Source: CAD feature listing. Evaluate the final solid. Frame: model axes, mm. Face numbers are marked on the shaded views. A direction names the side the tool comes from. Give positions to 0.01 mm unless a question says otherwise; leave off trailing zeros. Write each loop counter-clockwise with the first axis right and the second up, starting at its lowest first coordinate (ties: lowest second). Pieces come first, ordered by that corner, then holes. Notation, with made-up numbers: (31, 5.25) -> (51, 5.25) arc R24 ccw to (51, 26.25) -> close; hole circle Ø2 at (34.5, 43). An arc over 180 degrees is marked (long way). Answer as a JSON object with one key per item and string values. Group by question number.
Item 1: Section query A-A on x = -45. Return the cut outline in (y, z), plus the area to 3 significant figures.
Item 2: Access query for the marked faces 1 and 2. Directions: +Z, -Z, +X, -X, +Y, -Y. A direction counts if a zero-diameter tool reaches every point of the face in a straight line with its end or side. Return the directions, or none.
Item 3: Section query C-C on y = 2.25. Give the number of separate pieces and of enclosed holes in the cut face, plus the area to 3 significant figures.
Item 4: First-contact query: pin 1 Ø5.5 at (x, z) = (54.28, 54.28) entering from -Y; pin 2 Ø4.5 at (x, z) = (-54.28, 54.28) entering from +Y; pin 3 Ø2 at (y, z) = (0.5, 50) entering from +X. Flat tips, straight axial feed; report the tip coordinate or a pass-through.
Item 5: Section query B-B on z = -12.5. Return the cut outline in (x, y), plus the area to 3 significant figures.
Item 6: Ray query, probe 1 along X at (y, z) = (0.35, 0); probe 2 along Y at (x, z) = (-64.5, -46.5). Return the intervals inside material, ascending. Write a range as from..to.
from build123d import *
from build123d.topology import SkipClean

# Parameters (mm, degrees)
ESBO_O1_R                                    = 82.26
ESBO_O1_R_2                                  = 70
RESSALTO_EXTRUS_O1_DEPTH                     = 3
RESSALTO_EXTRUS_O2_START                     = 1.3
ESBO_O2_R                                    = 73
ESBO_O2_R_2                                  = 70
RESSALTO_EXTRUS_O2_DEPTH                     = 1.3
ESCAREADO_PARA_PARAFUSO_ALLEN_SEXTAV_2_COUNT = 2
ESCAREADO_PARA_PARAFUSO_ALLEN_SEXTAV_2_PITCH = 76.76
ESCAREADO_PARA_PARAFUSO_ALLEN_SEXTAV_3_COUNT = 2
ESCAREADO_PARA_PARAFUSO_ALLEN_SEXTAV_3_PITCH = 76.76
ESCAREADO_PARA_PARAFUSO_ALLEN_SEXTAV_4_COUNT = 2
ESCAREADO_PARA_PARAFUSO_ALLEN_SEXTAV_4_PITCH = 76.76
ESCAREADO_PARA_PARAFUSO_ALLEN_SEXTAV_5_COUNT = 2
ESCAREADO_PARA_PARAFUSO_ALLEN_SEXTAV_5_PITCH = 76.76
ESCAREADO_PARA_PARAFUSO_ALLEN_SEXTAV_6_COUNT = 2
ESCAREADO_PARA_PARAFUSO_ALLEN_SEXTAV_6_PITCH = 76.76
ESCAREADO_PARA_PARAFUSO_ALLEN_SEXTAV_7_COUNT = 2
ESCAREADO_PARA_PARAFUSO_ALLEN_SEXTAV_7_PITCH = 76.76
ESCAREADO_PARA_PARAFUSO_ALLEN_SEXTAV_8_COUNT = 2
ESCAREADO_PARA_PARAFUSO_ALLEN_SEXTAV_8_PITCH = 76.76
ESCAREADO_PARA_PARAFUSO_ALLEN_SEXTAV_9_COUNT = 2
ESCAREADO_PARA_PARAFUSO_ALLEN_SEXTAV_9_PITCH = 76.76
RESSALTO_EXTRUS_O3_START                     = -3
RESSALTO_EXTRUS_O3_DEPTH                     = 3
FILETE1_R                                    = 2
ESBO_O9_R                                    = 1.8
CORTE_EXTRUS_O3_DEPTH                        = 122.035496877
CHANFRO2_SIZE                                = 1


with BuildPart() as part:
    # Esboço1 → Ressalto-extrusão1 (new body)
    with BuildSketch(Plane(origin=(0, 0, 0), x_dir=(1, 0, 0), z_dir=(0, 1, 0))):
        with Locations(Location((0, 0, 0), (0, 0, 270))):
            Circle(ESBO_O1_R)
        with Locations(Location((0, 0, 0), (0, 0, 270))):
            Circle(ESBO_O1_R_2, mode=Mode.SUBTRACT)
    extrude(amount=RESSALTO_EXTRUS_O1_DEPTH)

    # Esboço2 → Ressalto-extrusão2 (add)
    with SkipClean():  # the faces are left unmerged after this step: merging them gives an invalid solid
        with BuildSketch(Plane.XZ.offset(RESSALTO_EXTRUS_O2_START)):
            with Locations(Location((0, 0, 0), (0, 0, 270))):
                Circle(ESBO_O2_R)
            with Locations(Location((0, 0, 0), (0, 0, 270))):
                Circle(ESBO_O2_R_2, mode=Mode.SUBTRACT)
        extrude(amount=-RESSALTO_EXTRUS_O2_DEPTH)

    # Esboço4 → Escareado para parafuso Allen sextavado escareado de M31 (revolve, cut)
    with SkipClean():  # the faces are left unmerged after this step: merging them gives an invalid solid
        with BuildSketch(Plane(origin=(0, 3, 0), x_dir=(0, 0, 1), z_dir=(1, 0, 0))):
            Polygon((0, 0), (0, 3), (1.7, 3), (1.7, 1.66), (3.36, 0), align=None)
        escareado_para_parafuso_allen_sextavado = revolve(axis=Axis((0, 9.35, 0), (0, -1, 0)), mode=Mode.SUBTRACT)

    # Escareado para parafuso Allen sextav 2: Escareado para parafuso Allen sextavado escareado de M31 ×2
    with SkipClean():  # the faces are left unmerged after this step: merging them gives an invalid solid
        with Locations(*[(-i * ESCAREADO_PARA_PARAFUSO_ALLEN_SEXTAV_2_PITCH, 0, 0) for i in range(1, ESCAREADO_PARA_PARAFUSO_ALLEN_SEXTAV_2_COUNT)]):
            add(escareado_para_parafuso_allen_sextavado, mode=Mode.SUBTRACT)

    # Escareado para parafuso Allen sextav 3: Escareado para parafuso Allen sextavado escareado de M31 ×2
    with SkipClean():  # the faces are left unmerged after this step: merging them gives an invalid solid
        with Locations(*[Vector(-0.7071067811865477, 0, -0.7071067811865475) * (i * ESCAREADO_PARA_PARAFUSO_ALLEN_SEXTAV_3_PITCH) for i in range(1, ESCAREADO_PARA_PARAFUSO_ALLEN_SEXTAV_3_COUNT)]):
            add(escareado_para_parafuso_allen_sextavado, mode=Mode.SUBTRACT)

    # Escareado para parafuso Allen sextav 4: Escareado para parafuso Allen sextavado escareado de M31 ×2
    with SkipClean():  # the faces are left unmerged after this step: merging them gives an invalid solid
        with Locations(*[(0, 0, -i * ESCAREADO_PARA_PARAFUSO_ALLEN_SEXTAV_4_PITCH) for i in range(1, ESCAREADO_PARA_PARAFUSO_ALLEN_SEXTAV_4_COUNT)]):
            add(escareado_para_parafuso_allen_sextavado, mode=Mode.SUBTRACT)

    # Escareado para parafuso Allen sextav 5: Escareado para parafuso Allen sextavado escareado de M31 ×2
    with SkipClean():  # the faces are left unmerged after this step: merging them gives an invalid solid
        with Locations(*[Vector(0.7071067811865475, 0, -0.7071067811865476) * (i * ESCAREADO_PARA_PARAFUSO_ALLEN_SEXTAV_5_PITCH) for i in range(1, ESCAREADO_PARA_PARAFUSO_ALLEN_SEXTAV_5_COUNT)]):
            add(escareado_para_parafuso_allen_sextavado, mode=Mode.SUBTRACT)

    # Escareado para parafuso Allen sextav 6: Escareado para parafuso Allen sextavado escareado de M31 ×2
    with SkipClean():  # the faces are left unmerged after this step: merging them gives an invalid solid
        with Locations(*[(i * ESCAREADO_PARA_PARAFUSO_ALLEN_SEXTAV_6_PITCH, 0, 0) for i in range(1, ESCAREADO_PARA_PARAFUSO_ALLEN_SEXTAV_6_COUNT)]):
            add(escareado_para_parafuso_allen_sextavado, mode=Mode.SUBTRACT)

    # Escareado para parafuso Allen sextav 7: Escareado para parafuso Allen sextavado escareado de M31 ×2
    with SkipClean():  # the faces are left unmerged after this step: merging them gives an invalid solid
        with Locations(*[Vector(0.7071067811865477, 0, 0.7071067811865475) * (i * ESCAREADO_PARA_PARAFUSO_ALLEN_SEXTAV_7_PITCH) for i in range(1, ESCAREADO_PARA_PARAFUSO_ALLEN_SEXTAV_7_COUNT)]):
            add(escareado_para_parafuso_allen_sextavado, mode=Mode.SUBTRACT)

    # Escareado para parafuso Allen sextav 8: Escareado para parafuso Allen sextavado escareado de M31 ×2
    with SkipClean():  # the faces are left unmerged after this step: merging them gives an invalid solid
        with Locations(*[(0, 0, i * ESCAREADO_PARA_PARAFUSO_ALLEN_SEXTAV_8_PITCH) for i in range(1, ESCAREADO_PARA_PARAFUSO_ALLEN_SEXTAV_8_COUNT)]):
            add(escareado_para_parafuso_allen_sextavado, mode=Mode.SUBTRACT)

    # Escareado para parafuso Allen sextav 9: Escareado para parafuso Allen sextavado escareado de M31 ×2
    with SkipClean():  # the faces are left unmerged after this step: merging them gives an invalid solid
        with Locations(*[Vector(-0.7071067811865475, 0, 0.7071067811865476) * (i * ESCAREADO_PARA_PARAFUSO_ALLEN_SEXTAV_9_PITCH) for i in range(1, ESCAREADO_PARA_PARAFUSO_ALLEN_SEXTAV_9_COUNT)]):
            add(escareado_para_parafuso_allen_sextavado, mode=Mode.SUBTRACT)

    # Esboço5 → Ressalto-extrusão3 (add)
    with SkipClean():  # the faces are left unmerged after this step: merging them gives an invalid solid
        with BuildSketch(Plane(origin=(0, 3, 0), x_dir=(1, 0, 0), z_dir=(0, 1, 0)).offset(RESSALTO_EXTRUS_O3_START)):
            with BuildLine():
                Line((59.628675028, -61.836305796), (71.511245178, -82.577126452))
                ThreePointArc((71.511245178, -82.577126452), (81.110607536, -73.170413044), (89.482153659, -62.656078528))
                Line((89.482153659, -62.656078528), (67.383447163, -47.182397654))
                ThreePointArc((67.383447163, -47.182397654), (62.829570926, -53.09569302), (57.758469462, -58.57189433))
                Line((57.758469462, -58.57189433), (59.628675028, -61.836305796))
            make_face()
        extrude(amount=RESSALTO_EXTRUS_O3_DEPTH)
    add(part.part.scale(1), mode=Mode.REPLACE)  # the faces are merged on a copy

    # Filete1
    # the kernel refuses this fillet: 2 mm, written as the material it adds along each edge
    with BuildSketch(Plane(origin=(57.758469462, 0, 58.57189433), x_dir=(-0.7227263558173935, 0, 0.6911342956379103), z_dir=(0, 1, 0))) as filete1_piece_1:
        with BuildLine():
            CenterArc((2.55574236, 1.999764426), FILETE1_R, 166.088750143, 103.031841977)
            Line((0.61440377, 2.480601697), (0, 0))
            ThreePointArc((0, 0), (1.26252322, 0.009689149), (2.525046439, 0))
        make_face()
    extrude(amount=3)
    with BuildSketch(Plane(origin=(67.383447163, 0, 47.182397654), x_dir=(0.5638136312570139, 0, -0.8259020457710344), z_dir=(0, 1, 0))) as filete1_piece_2:
        with BuildLine():
            CenterArc((1.976403158, -1.999859125), FILETE1_R, 90.680051756, 88.639896488)
            Line((-0.023455967, -1.976121398), (0, 0))
            ThreePointArc((0, 0), (0.976332715, -0.005794184), (1.952665431, 0))
        make_face()
    extrude(amount=3)
    # the kernel refuses this fillet: 2 mm, written as the material it takes off along each edge
    with BuildSketch(Plane(origin=(89.482153659, -5.093472409, 62.656078528), x_dir=(-0.5811904962497088, 0, 0.8137675387166886), z_dir=(0, 1, 0))) as filete1_2_piece_1:
        with BuildLine():
            CenterArc((2.018737967, -1.999913033), FILETE1_R, 89.465680564, 91.068638872)
            Line((0.018824934, -2.01856403), (0, 0))
            ThreePointArc((0, 0), (1.018694482, 0.00475002), (2.037388964, 0))
        make_face()
    extrude(amount=13.186944818, mode=Mode.SUBTRACT)
    with BuildSketch(Plane(origin=(71.511245178, -6.20199849, 82.577126452), x_dir=(-0.4971059552935667, 0, -0.8676898462075434), z_dir=(0, 1, 0))) as filete1_2_piece_2:
        with BuildLine():
            CenterArc((2.457984349, -2), FILETE1_R, 90, 102.384853671)
            ThreePointArc((0.504526328, -2.428954266), (0.245367707, -1.215909412), (0, 0))
            Line((0, 0), (2.457984349, 0))
        make_face()
    extrude(amount=15.40399698, mode=Mode.SUBTRACT)

    # Esboço9 → Corte-extrusão3 (cut, through all)
    with BuildSketch(Plane(origin=(0, 3, 0), x_dir=(1, 0, 0), z_dir=(0, 1, 0))):
        with Locations(Location((75.866996657, -59.226515904, 0), (0, 0, 270))):
            Circle(ESBO_O9_R)
    extrude(amount=-CORTE_EXTRUS_O3_DEPTH, mode=Mode.SUBTRACT)

    # Chanfro2
    chanfro2_edges = [part.edges().sort_by_distance(p)[0] for p in [
        (75.866996657, 0, 57.426515904),
    ]]
    chamfer(chanfro2_edges, length=CHANFRO2_SIZE)


solid = part.part
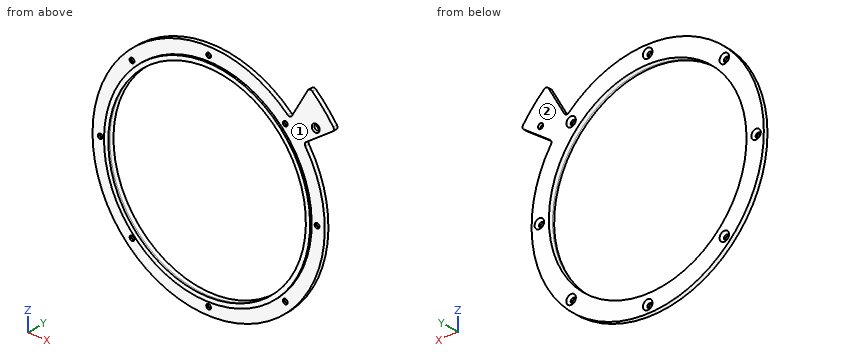
Worked answers:
{
 "1": {"outline": "(-1.3, -57.48) -> (0, -57.48) -> (0, -68.86) -> (3, -68.86) -> (3, -53.62) -> (-1.3, -53.62) -> close; (-1.3, 53.62) -> (3, 53.62) -> (3, 68.86) -> (0, 68.86) -> (0, 57.48) -> (-1.3, 57.48) -> close", "area": "101 mm^2"},
 "2": {"face 1": "-Y", "face 2": "+Z, -Z, +X, -X, +Y"},
 "3": {"separate pieces": "1", "enclosed holes": "10", "area": "6,250 mm^2"},
 "4": {"pin 1": "y = 0", "pin 2": "y = 1.89", "pin 3": "x = 72.84"},
 "5": {"outline": "(-81.3, 0) -> (-71.92, 0) -> (-71.92, -1.3) -> (-68.87, -1.3) -> (-68.87, 3) -> (-81.3, 3) -> close; (68.87, -1.3) -> (71.92, -1.3) -> (71.92, 0) -> (81.3, 0) -> (81.3, 3) -> (68.87, 3) -> close", "area": "82.5 mm^2"},
 "6": {"probe 1": "-82.26..-78.46, -75.06..-70, 70..75.06, 78.46..82.26", "probe 2": "0..3"}
}
